Design review of the part built by this model. Coordinates are the model's own, in mm. A direction names the side the tool comes from. Round coordinates to 2 decimals unless told otherwise and drop trailing zeros. Order: outer loops, then holes, each group sorted by start corner. A loop starts at its lowest first (then second) coordinate and runs counter-clockwise, first axis right, second up. Notation, with made-up numbers: (55.25, 40.25) - (105.25, 40.25) arc R24 cw to (105.25, 70.25) - close; hole circle Ø8 at (77.25, 23.25). An arc over 180 degrees is marked (long way). Write item = value, one per line.
Autodesk Inventor part; units mm, degrees
ref_plane "YZ Plane" through (0, 0, 0) normal (1, 0, 0) x (0, 1, 0)
ref_plane "XZ Plane" through (0, 0, 0) normal (0, 1, 0) x (-1, 0, 0)
ref_plane "XY Plane" through (0, 0, 0) normal (0, 0, 1) x (1, 0, 0)
sketch "スケッチ1" plane through (0, 0, 0) normal (0, 0, 1) x (1, 0, 0)
  circle A0 centre (0, 0) radius 1.5
  dimension "d0" = 3
extrude "押し出し1" add sketch "スケッチ1" along normal blind 6
sketch "スケッチ2" plane through (0, 0, 0) normal (0, 0, -1) x (-1, 0, 0)
  circle A0 centre (0, 0) radius 2.75
  dimension "d3" = 5.5
extrude "押し出し2" add sketch "スケッチ2" along normal blind 2
fillet "フィレット1" radius 2 1 edges at (2.75, 0, -2)
thread "ねじ1"
properties part number "ネジ鍋m3,06" material "鋼、高強度、低合金"
1) For faces 1 (the flat face through (0, 0, -2)), 2 (the flat face through (-1.2, -1.2, 0)), list the 3-axis set-ups (+Z, -Z, +X, -X, +Y, -Y) from which the entire face can be reached by the end or side of a thin tool; tool diameter is ignored.
Findings:
face_1 = -Z, +X, -X, +Y, -Y
face_2 = +Z
2) Clearance check with flat-ended pins moving along their axes: pin 1 Ø3 at (y, z) = (0.5, -0.5) entering from +X; pin 2 Ø2 at (y, z) = (-0.5, 3.5) entering from +X; pin 3 Ø2 at (x, z) = (2, 4) entering from -Y. State where each tip first meets the part, or that it passes through.
Findings:
pin_1 = 2.75
pin_2 = 1.5
pin_3 = -1.12
3) We need section A-A on z = 5. Write out the cut boundary in (x, y).
Findings:
outline = circle Ø3 at (0, 0)
4) To check wall thickness, follow L1, parallel to X at y = -0.05, z = 0.5; L2, parallel to Y at x = 1.05, z = 2; L3, parallel to X at y = 0.4, z = 0.5. State the ranges of each line that lie inside material, in increasing order. Write a range as from..to.
Findings:
L1 = -1.5..1.5
L2 = -1.07..1.07
L3 = -1.45..1.45
